Read the model definition and answer for the solid it produces. Units are mm, in the model's axes. A direction names the side the tool comes from. Coordinates: 2 decimals unless noted, no trailing zeros. Write each loop counter-clockwise with the first axis right and the second up, starting at its lowest first coordinate (ties: lowest second). Pieces come first, ordered by that corner, then holes. Notation, with made-up numbers: M 31,12.5 L 68,12.5 A24 ccw 68,31.5 Z; hole C 7,53.5 d2. An arc over 180 degrees is marked long. Write item = value, one per line.
from build123d import *

# Parameters (mm, degrees)
SKETCH_1_R          = 30
SKETCH_1_R_2        = 5
EXTRUDE_1_DEPTH     = 10
SKETCH_3_W          = 40
SKETCH_3_H          = 24
EXTRUDE_2_DEPTH     = 30
SKETCH_4_R          = 20
CUT_EXTRUDE_2_DEPTH = 71.710678119


with BuildPart() as part:
    # 草图1 → 凸台-拉伸1 (new body)
    with BuildSketch(Plane(origin=(0, 0, 0), x_dir=(0, 0, -1), z_dir=(1, 0, 0))):
        Circle(SKETCH_1_R)
        Circle(SKETCH_1_R_2, mode=Mode.SUBTRACT)
    extrude(amount=EXTRUDE_1_DEPTH)

    # 草图3 → 凸台-拉伸2 (add)
    with BuildSketch(Plane(origin=(10, 0, 0), x_dir=(0, 0, -1), z_dir=(1, 0, 0))):
        Rectangle(SKETCH_3_W, SKETCH_3_H)
    extrude(amount=EXTRUDE_2_DEPTH)

    # 草图4 → 切除-拉伸2 (cut, through all)
    with BuildSketch(Plane(origin=(0, 0, -20), x_dir=(-1, 0, 0), z_dir=(0, 0, -1))):
        with Locations((-50, 0)):
            Circle(SKETCH_4_R)
    extrude(amount=-CUT_EXTRUDE_2_DEPTH, mode=Mode.SUBTRACT)


solid = part.part
Item 1: Flat-ended cylindrical pins translate along their axes: pin 1 (8 mm diameter, centred on y = -17, z = 8, fed in from +X); pin 2 (5 mm diameter, centred on x = 15.5, z = -21, fed in from -Y); pin 3 (7 mm diameter, centred on x = 23, z = 10, fed in from +Y). Find the tip coordinate at first contact, or state that the pin passes through.
Worked answers:
pin_1 = 10
pin_2 = -12
pin_3 = 12
Item 2: Consider line 1 along Y through (x, z) = (2, 0); line 2 along Y through (x, z) = (20.5, -3.5); line 3 along X through (y, z) = (-15.5, -15). Determine where each line is inside the solid, lowest interval first. Write a range as from..to.
Worked answers:
line_1 = -30..-5, 5..30
line_2 = -12..12
line_3 = 0..10
Item 3: Find section C-C (x = 2.5). Determine the outline of the cut face in (y, z), and give its area (3 significant figures).
Worked answers:
outline = C 0,0 d60; hole C 0,0 d10
area = 2,750 mm²
Item 4: Which of the six approach directions +Z, -Z, +X, -X, +Y, -Y give full straight-line access (tool end or side, diameter ignored) to faces 1 (the face through (30, 0, 0)), 2 (the face through (22, 12, 0)), 3 (the face through (22, -12, 0)), 4 (the face through (22, 0, -20)), 5 (the face through (22, 0, 20))?
Worked answers:
face_1 = +Z, -Z, +X
face_2 = +Z, -Z, +X, +Y
face_3 = +Z, -Z, +X, -Y
face_4 = -Z, +X, +Y, -Y
face_5 = +Z, +X, +Y, -Y
Item 5: Find section A-A (y = 0). Determine the outline of the cut face in (x, z), and give its area (3 significant figures).
Worked answers:
outline = M 0,-30 L 10,-30 L 10,-20 L 30,-20 L 30,20 L 10,20 L 10,30 L 0,30 L 0,5 L 10,5 L 10,-5 L 0,-5 Z
area = 1,300 mm²
Item 6: Find section D-D (x = 21.5). Determine the outline of the cut face in (y, z), and give its area (3 significant figures).
Worked answers:
outline = M -12,-20 L 12,-20 L 12,20 L -12,20 Z
area = 960 mm²
Item 7: For a pull along Y with two mould halves and no side action, classify faces 6 (the face through (10, 0, 0)), 7 (the face through (0, 0, -6)), 8 (the face through (4.93, 1.32, 29.97)), 9 (the face through (4.93, -4.88, 1.08)) as released by +Y, released by -Y, zero draft, split by the parting line, or undercut.
Worked answers:
face_6 = undercut
face_7 = zero draft
face_8 = split by the parting line
face_9 = undercut
Item 8: Find section B-B (z = 0). Determine the outline of the cut face in (x, y).
Worked answers:
outline = M 0,-30 L 10,-30 L 10,-12 L 34,-12 A20 cw 34,12 L 10,12 L 10,30 L 0,30 L 0,5 L 10,5 L 10,-5 L 0,-5 Z
